from build123d import *

# Parameters (mm, degrees)
SKETCH1_W               = 13
SKETCH1_H               = 8
BOSS_EXTRUDE1_DEPTH     = 3
CUT_EXTRUDE1_DEPTH      = 16.556349186
CUT_EXTRUDE1_DEPTH_BACK = 16.556349186
CUT_EXTRUDE2_DEPTH      = 16.556349186
CUT_EXTRUDE2_DEPTH_BACK = 16.556349186
SKETCH4_R               = 1.75
CUT_EXTRUDE3_DEPTH      = 0.4
SKETCH5_W               = 8
SKETCH5_H               = 1.1
BOSS_EXTRUDE2_DEPTH     = 2
FILLET1_R               = 4
SKETCH6_W               = 0.576923077
SKETCH6_H               = 3
CUT_EXTRUDE4_DEPTH      = 0.4


with BuildPart() as part:
    # Sketch1 → Boss-Extrude1 (new body)
    with BuildSketch(Plane(origin=(0, 0, 0), x_dir=(1, 0, 0), z_dir=(0, 1, 0))):
        with Locations((6.5, 4)):
            Rectangle(SKETCH1_W, SKETCH1_H)
    extrude(amount=BOSS_EXTRUDE1_DEPTH)

    # Sketch2 → Cut-Extrude1 (cut, two sides: drawn at the far end of the back side and taken through both)
    with BuildSketch(Plane.XY.offset(-CUT_EXTRUDE1_DEPTH_BACK)):
        Polygon((0, 0), (0.6, 3), (0, 3), align=None)
        Polygon((13, 0), (12.4, 3), (13, 3), align=None)
    extrude(amount=CUT_EXTRUDE1_DEPTH + CUT_EXTRUDE1_DEPTH_BACK, mode=Mode.SUBTRACT)

    # Sketch3 → Cut-Extrude2 (cut, two sides: drawn at the far end of the back side and taken through both)
    with BuildSketch(Plane(origin=(0, 0, 0), x_dir=(0, 0, -1), z_dir=(1, 0, 0)).offset(-CUT_EXTRUDE2_DEPTH_BACK)):
        Polygon((0, 0), (0.6, 3), (0, 3), align=None)
        Polygon((8, 3), (7.4, 3), (8, 0), align=None)
    extrude(amount=CUT_EXTRUDE2_DEPTH + CUT_EXTRUDE2_DEPTH_BACK, mode=Mode.SUBTRACT)

    # Sketch4 → Cut-Extrude3 (cut)
    with BuildSketch(Plane.XZ):
        with Locations(Location((6.50000125, -3.75, 0), (0, 0, 270))):
            Circle(SKETCH4_R)
    extrude(amount=-CUT_EXTRUDE3_DEPTH, mode=Mode.SUBTRACT)

    # Sketch5 → Boss-Extrude2 (add)
    with BuildSketch(Plane.XZ):
        with Locations((6.500011, -7.45)):
            Rectangle(SKETCH5_W, SKETCH5_H)
    extrude(amount=BOSS_EXTRUDE2_DEPTH)

    # Fillet1
    # the kernel refuses this fillet: 4 mm, written as the material it takes off along each edge
    with BuildSketch(Plane(origin=(10.500011, -2, -16.660254038), x_dir=(0, 1, 0), z_dir=(0, 0, 1)), Plane(origin=(2.500011, -2, 1.760254038), x_dir=(0, 1, 0), z_dir=(0, 0, -1))) as fillet1_piece_1:
        with BuildLine():
            CenterArc((4, 3.464101615), FILLET1_R, 180, 60)
            Line((0, 3.464101615), (-0.08, 3.464101615))
            Line((-0.08, 3.464101615), (-0.08, 0))
            Line((-0.08, 0), (0, -0.08))
            ThreePointArc((0, -0.08), (1, -0.08), (1.96, -0.069282032))
            Line((1.96, -0.069282032), (2, 0))
        make_face()
    extrude(amount=18.420508076, mode=Mode.SUBTRACT)

    # Sketch6 → Cut-Extrude4 (cut)
    with BuildSketch(Plane(origin=(0, 3, 0), x_dir=(1, 0, 0), z_dir=(0, 1, 0))):
        Polygon((3.219165588, 2.557267472), (2.50101655, 5.557267472), (3.092362704, 5.557267472), (3.558708858, 3.496570357), (4.052098281, 5.557267472), (4.839357896, 5.557267472), (5.327939627, 3.461714587), (5.793083858, 5.557267472), (6.385631934, 5.557267472), (5.68070405, 2.557267472), (4.966160781, 2.557267472), (4.443324242, 4.800055934), (3.906665588, 2.557267472), align=None)
        with Locations((6.981785781, 4.057267472)):
            Rectangle(SKETCH6_W, SKETCH6_H)
        Polygon((7.885631934, 2.557267472), (7.885631934, 5.557267472), (8.488396358, 5.557267472), (9.693324242, 3.584911703), (9.693324242, 5.557267472), (10.270247319, 5.557267472), (10.270247319, 2.557267472), (9.648853088, 2.557267472), (8.462555011, 4.498373241), (8.462555011, 2.557267472), align=None)
    extrude(amount=-CUT_EXTRUDE4_DEPTH, mode=Mode.SUBTRACT)


solid = part.part
Model file for the job. Use its own axes, mm. A direction names the side the tool comes from. Give positions to 0.01 mm unless a question says otherwise; leave off trailing zeros. Loops run counter-clockwise (first coordinate to the right, second up) from the corner with the lowest first, then second, coordinate; pieces in that order, holes last. Notation, with made-up numbers: (-4, 26.25) - (32, 26.25) arc R20 cw to (32, 43.25) - close; hole circle Ø11 at (-7, -31). An arc over 180 degrees is marked (long way). Use one line per item in the form item = value.
(1) Cut at A-A (x = 6.25). Give the cut face in (y, z).
Determined:
outline = (-2, -8) - (0, -8) - (3, -7.4) - (3, -5.56) - (2.6, -5.56) - (2.6, -4.98) - (3, -4.98) - (3, -0.6) - (0, 0) - (0, -2.02) - (0.4, -2.02) - (0.4, -5.48) - (0, -5.48) - (0, -6.9) - (-2, -6.9) - close
(2) Drop flat-ended pins along their axis: P1, Ø1.6, axis at x = 8, y = -1, coming from the +Z side; P2, Ø3, axis at x = 7, z = -3.5, coming from the -Y side; P3, Ø3, axis at y = 2, z = -5.5, coming from the +X side. Give the stop position or say it passes through.
Determined:
P1 = -6.9
P2 = 0
P3 = 12.9
(3) Cut at B-B (z = -1.25). Give the cut face in (x, y), then the cut area to 3 significant figures.
Determined:
outline = (0, 0) - (13, 0) - (12.4, 3) - (0.6, 3) - close
area = 37.2 mm^2
(4) Cut at C-C (y = 1.05). Give the cut face in (x, z), then the cut area to 3 significant figures.
Determined:
outline = (0.21, -7.79) - (12.79, -7.79) - (12.79, -0.21) - (0.21, -0.21) - close
area = 95.4 mm^2
(5) 3-axis set-ups, long thin cutter, end or side, ignore diameter. For faces 1 (the face through (6, -1, -6.9)), 2 (the face through (9.064, 2.803, -3.514)), 3 (the face through (7, 0.4, -4)), 4 (the face through (6.4, 3, -4)): which of +Z, -Z, +X, -X, +Y, -Y reach the whole face in a straight line?
Determined:
face_1 = +Z, +X, -X, -Y
face_2 = +Y
face_3 = -Y
face_4 = +Z, -Z, +X, -X, +Y
(6) Drill centre lines: L1, parallel to Y at x = 5, z = -4.25; L2, parallel to Y at x = 11.75, z = -6.5; L3, parallel to X at y = 0.2, z = -3.75. Where is each one in solid material? Low to high.
Determined:
L1 = 0.4 to 2.6
L2 = 0 to 3
L3 = 0.04 to 4.75, 8.25 to 12.96
(7) Pull direction X, two halves, no side cores. Call faces 5 (the face through (3.99, -1.48, -7.44)), 6 (the face through (9.082, 2.803, -4.585)), 7 (the face through (6.5, -2, -7.4)), 8 (the face through (12.7, 1.5, -4.1)): pulls with the +X half, pulls with the -X half, needs draft (parallel to the pull), parting line crosses it, or undercut.
Determined:
face_5 = pulls with the -X half
face_6 = undercut
face_7 = needs draft
face_8 = pulls with the +X half
